from build123d import *

# Parameters (mm, degrees)
SKETCH1_R             = 15.24
SKETCH1_R_2           = 4.55
BOSS_EXTRUDE1_DEPTH   = 2.54
SKETCH2_R             = 5.95
BOSS_EXTRUDE2_DEPTH   = 19.05
SKETCH5_R             = 1.27
BOSS_EXTRUDE5_DEPTH   = 4.000000128
M5X0_8_TAPPED_HOLE2_D = 4.2


with BuildPart() as part:
    # Sketch1 → Boss-Extrude1 (new body)
    with BuildSketch(Plane.XY):
        Circle(SKETCH1_R)
        Circle(SKETCH1_R_2, mode=Mode.SUBTRACT)
    extrude(amount=BOSS_EXTRUDE1_DEPTH)

    # Sketch2 → Boss-Extrude2 (add)
    with BuildSketch(Plane.XY.offset(2.54)):
        with Locations(Location((0, 0, 0), (0, 0, 180))):
            Circle(SKETCH2_R)
    extrude(amount=BOSS_EXTRUDE2_DEPTH)

    # Sketch5 → Boss-Extrude5 (add)
    with BuildSketch(Plane(origin=(0, 0, 0), x_dir=(-1, 0, 0), z_dir=(0, 0, -1))):
        with Locations(Location((0, 12.7, 0), (0, 0, 180))):
            Circle(SKETCH5_R)
        with Locations(Location((5.165555367, 11.602027312, 0), (0, 0, 180))):
            Circle(SKETCH5_R)
        with Locations(Location((9.437939284, 8.497958701, 0), (0, 0, 180))):
            Circle(SKETCH5_R)
        with Locations(Location((12.078417757, 3.924515829, 0), (0, 0, 180))):
            Circle(SKETCH5_R)
        with Locations(Location((12.630428071, -1.327511483, 0), (0, 0, 180))):
            Circle(SKETCH5_R)
        with Locations(Location((10.998522628, -6.35, 0), (0, 0, 180))):
            Circle(SKETCH5_R)
        with Locations(Location((7.464872704, -10.274515829, 0), (0, 0, 180))):
            Circle(SKETCH5_R)
        with Locations(Location((2.640478473, -12.422474529, 0), (0, 0, 180))):
            Circle(SKETCH5_R)
        with Locations(Location((-2.640478473, -12.422474529, 0), (0, 0, 180))):
            Circle(SKETCH5_R)
        with Locations(Location((-7.464872704, -10.274515829, 0), (0, 0, 180))):
            Circle(SKETCH5_R)
        with Locations(Location((-10.998522628, -6.35, 0), (0, 0, 180))):
            Circle(SKETCH5_R)
        with Locations(Location((-12.630428071, -1.327511483, 0), (0, 0, 180))):
            Circle(SKETCH5_R)
        with Locations(Location((-12.078417757, 3.924515829, 0), (0, 0, 180))):
            Circle(SKETCH5_R)
        with Locations(Location((-9.437939284, 8.497958701, 0), (0, 0, 180))):
            Circle(SKETCH5_R)
        with Locations(Location((-5.165555367, 11.602027312, 0), (0, 0, 180))):
            Circle(SKETCH5_R)
    extrude(amount=BOSS_EXTRUDE5_DEPTH)

    # M5x0.8 Tapped Hole2 (through all)
    with Locations(Plane.XY.offset(21.59)):
        with Locations((0, 0)):
            Hole(M5X0_8_TAPPED_HOLE2_D / 2)


solid = part.part
Source: CAD feature listing. Evaluate the final solid. Frame: model axes, mm. A direction names the side the tool comes from. Coordinates: 2 decimals unless noted, no trailing zeros. Write each loop counter-clockwise with the first axis right and the second up, starting at its lowest first coordinate (ties: lowest second). Pieces come first, ordered by that corner, then holes. Notation, with made-up numbers: M -32,-24.5 L -2,-24.5 A26 cw -2,13.5 Z; hole C 26.5,-4 d7. An arc over 180 degrees is marked long. Use a Markdown table: item, result.
1) Section A-A, the plane x = 0. Output: boundary loops of the cut face in (y, z).
Conclusion:
| item | result |
|---|---|
| outline | M -15.24,0 L -4.55,0 L -4.55,2.54 L -2.1,2.54 L -2.1,21.59 L -5.95,21.59 L -5.95,2.54 L -15.24,2.54 Z; M 2.1,2.54 L 4.55,2.54 L 4.55,0 L 11.43,0 L 11.43,-4 L 13.97,-4 L 13.97,0 L 15.24,0 L 15.24,2.54 L 5.95,2.54 L 5.95,21.59 L 2.1,21.59 Z |
2) Mould query, pull axis X, two halves, no side actions, for faces 3 (the flat face through (-13, -1, -4)), 4 (the cylindrical face through (0.586, 13.827, -1.972)). Classes: pulls with the +X half, pulls with the -X half, needs draft (parallel to the pull), parting line crosses it, or undercut.
Conclusion:
| item | result |
|---|---|
| face 3 | needs draft |
| face 4 | undercut |
3) First-contact query: pin 1 Ø5 at (x, z) = (5.5, 11) entering from -Y; pin 2 Ø8 at (y, z) = (-0.5, 10) entering from -X; pin 3 Ø3 at (y, z) = (-5.5, 14.5) entering from +X. Flat tips, straight axial feed; report the tip coordinate or a pass-through.
Conclusion:
| item | result |
|---|---|
| pin 1 | stops at y = -5.14 |
| pin 2 | stops at x = -5.95 |
| pin 3 | stops at x = 4.4 |
4) Section C-C, the plane x = -5. Output: boundary loops of the cut face in (y, z).
Conclusion:
| item | result |
|---|---|
| outline | M -14.4,0 L 10.34,0 L 10.34,-4 L 12.86,-4 L 12.86,0 L 14.4,0 L 14.4,2.54 L 3.23,2.54 L 3.23,21.59 L -3.23,21.59 L -3.23,2.54 L -14.4,2.54 Z |
5) Ray query, L1, parallel to Y at x = 0, z = 6.75; L2, parallel to Z at x = 8.5, y = -3.5; L3, parallel to Y at x = 0, z = 1.1. Return the intervals inside material, ascending.
Conclusion:
| item | result |
|---|---|
| L1 | y = -5.95 to -2.1, 2.1 to 5.95 |
| L2 | z = 0 to 2.54 |
| L3 | y = -15.24 to -4.55, 4.55 to 15.24 |
6) Section B-B, the plane z = 7.25. Output: boundary loops of the cut face in (x, y), then the cut area to 3 significant figures.
Conclusion:
| item | result |
|---|---|
| outline | C 0,0 d11.9; hole C 0,0 d4.2 |
| area | 97.4 mm^2 |
7) Reachability of faces 1 (the flat face through (12, 4, -4)), 2 (the cylindrical face through (-2.916, -11.183, -1.972)) from +Z, -Z, +X, -X, +Y, -Y: full face, straight path, thin tool, end or side. Return the list, or none.
Conclusion:
| item | result |
|---|---|
| face 1 | -Z, +X, -X, +Y, -Y |
| face 2 | -Z |
